from build123d import *

# Parameters (mm, degrees)
BOSS_EXTRUDE1_DEPTH = 3
SKETCH3_W           = 21
SKETCH3_H           = 6
CUT_EXTRUDE1_DEPTH  = 10


with BuildPart() as part:
    # Sketch2 → Boss-Extrude1 (new body)
    with BuildSketch(Plane.XY):
        Polygon((0, 0), (77, 0), (77, 47.04888), (65.6794, 66.86939), (43.56615, 66.86939), (36.71335, 55), (0, 55), align=None)
    extrude(amount=BOSS_EXTRUDE1_DEPTH)

    # Sketch3 → Cut-Extrude1 (cut)
    with BuildSketch(Plane(origin=(0, 0, 0), x_dir=(-1, 0, 0), z_dir=(0, 0, -1))):
        with Locations((-52, 27.41)):
            Rectangle(SKETCH3_W, SKETCH3_H)
    extrude(amount=-CUT_EXTRUDE1_DEPTH, mode=Mode.SUBTRACT)


solid = part.part
Could you check a few things on this model? Use its own coordinates, in mm. A direction names the side the tool comes from. Coordinates: 2 decimals unless noted, no trailing zeros. Loops run counter-clockwise (first coordinate to the right, second up) from the corner with the lowest first, then second, coordinate; pieces in that order, holes last. Notation, with made-up numbers: (12.5, 70.5) -> (33.5, 70.5) arc R20 ccw to (33.5, 88.5) -> close; hole circle Ø11 at (69, -34.5). An arc over 180 degrees is marked (long way). Answer in a Markdown table with one row per item.
(1) Will these pins go through, and if not, where does the flat tip stop? pin 1 Ø1 at (x, z) = (42.5, 1) entering from +Y; pin 2 Ø1.5 at (x, z) = (67.5, 1.5) entering from +Y.
Results found:
| item | result |
|---|---|
| pin 1 | stops at y = 65.89 |
| pin 2 | stops at y = 64.99 |
(2) Imagine slicing it at C-C (x = 32). List the corners of the cut face in (y, z) for me.
Results found:
| item | result |
|---|---|
| outline | (0, 0) -> (55, 0) -> (55, 3) -> (0, 3) -> close |
(3) Imagine slicing it at A-A (z = 1.6). List the corners of the cut face in (x, y) for me.
Results found:
| item | result |
|---|---|
| outline | (0, 0) -> (77, 0) -> (77, 47.05) -> (65.68, 66.87) -> (43.57, 66.87) -> (36.71, 55) -> (0, 55) -> close; hole (41.5, 24.41) -> (62.5, 24.41) -> (62.5, 30.41) -> (41.5, 30.41) -> close |
(4) Thinking about a two-plate mould opening in X: for faces 4 (the face through (41.5, 27, 1)), 5 (the face through (38, 0, 1)), 6 (the face through (52, 24.41, 1)), 7 (the face through (77, 23, 1)), which applies, released by +X, released by -X, zero draft, split by the parting line, or undercut?
Results found:
| item | result |
|---|---|
| face 4 | undercut |
| face 5 | zero draft |
| face 6 | undercut |
| face 7 | released by +X |
(5) For faces 1 (the face through (19, 55, 1)), 2 (the face through (52, 30.41, 1)), 3 (the face through (38, 26, 0)), which set-ups out of +Z, -Z, +X, -X, +Y, -Y let a thin tool reach every point of the face, with its end or its side?
Results found:
| item | result |
|---|---|
| face 1 | +Z, -Z, -X, +Y |
| face 2 | +Z, -Z |
| face 3 | -Z, +X, -X, +Y, -Y |
(6) If I drill on probe 1 along Y at (x, z) = (57, 2.3); probe 2 along Y at (x, z) = (13, 1.25); probe 3 along Y at (x, z) = (40, 1.95), over which ranges is the centre line in solid material (lowest first)?
Results found:
| item | result |
|---|---|
| probe 1 | y = 0 to 24.41, 30.41 to 66.87 |
| probe 2 | y = 0 to 55 |
| probe 3 | y = 0 to 60.69 |
(7) Imagine slicing it at B-B (x = 53.5). List the corners of the cut face in (y, z) for me, plus the area to 3 significant figures.
Results found:
| item | result |
|---|---|
| outline | (0, 0) -> (24.41, 0) -> (24.41, 3) -> (0, 3) -> close; (30.41, 0) -> (66.87, 0) -> (66.87, 3) -> (30.41, 3) -> close |
| area | 183 mm^2 |
